For this review, use the dimensioned drawing (mm, ordinates from the lowest corner) and the shaded views. A direction names the side the tool comes from. Coordinates: 2 decimals unless noted, no trailing zeros. Loops run counter-clockwise (first coordinate to the right, second up) from the corner with the lowest first, then second, coordinate; pieces in that order, holes last. Notation, with made-up numbers: (-37.75, 16) - (-12.75, 16) arc R29 cw to (-12.75, 55) - close; hole circle Ø9 at (42, -27.75). An arc over 180 degrees is marked (long way). Answer in a Markdown table with one row per item. Add a question column.
(1) We need section B-B on y = 56.5. Write out the cut boundary in (x, z).
(2) For P1, Ø3, axis at x = 840.5, y = 23, coming from the +Z side; P2, Ø5.5, axis at x = 1167.96, z = 45, coming from the +Y side; P3, Ø3, axis at x = 295, z = 62, coming from the -Y side, all flat-tipped, find the tip position at first contact; note any pin that passes through.
(3) We need section C-C on z = 24. Write out the cut boundary in (x, y).
(4) Machinability: for the marked faces 1 and 2, which of the approach directions +Z, -Z, +X, -X, +Y, -Y give a long, thin tool a straight path to every point of the face, cutting with its end or side? Answer none if there is none.
(5) For line 1 along X through (y, z) = (36, 9) (1 decimal); line 2 along Y through (x, z) = (1161.08, 7) (3 decimals); line 3 along Y through (x, z) = (868, 11), list the stretches that pass through material, from the lowest coordinate up.
(6) We need section A-A on x = 384. Write out the cut boundary in (y, z).
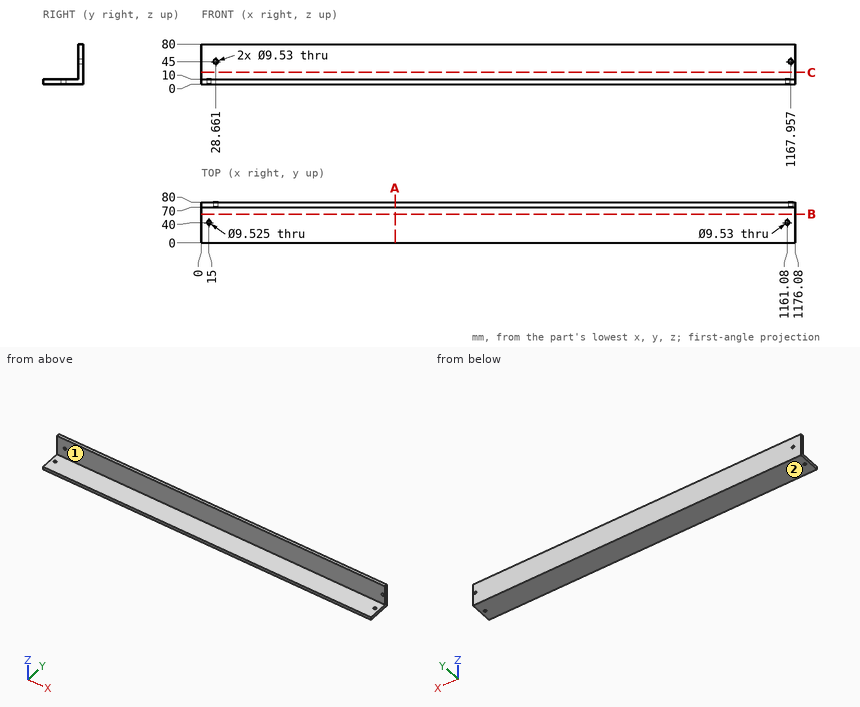
Outcome:
| question | item | result |
|---|---|---|
| 1 | outline | (0, 0) - (1176.08, 0) - (1176.08, 10) - (0, 10) - close |
| 2 | P1 | z = 10 |
| 2 | P2 | through |
| 2 | P3 | y = 70 |
| 3 | outline | (0, 70) - (1176.08, 70) - (1176.08, 80) - (0, 80) - close |
| 4 | face 1 | +Z, +X, -X, -Y |
| 4 | face 2 | -Z, +X, -X, +Y, -Y |
| 5 | line 1 | 0 to 12.4, 17.6 to 1158.5, 1163.7 to 1176.1 |
| 5 | line 2 | 0 to 35.235, 44.765 to 80 |
| 5 | line 3 | 70 to 80 |
| 6 | outline | (0, 0) - (80, 0) - (80, 80) - (70, 80) - (70, 10) - (0, 10) - close |
